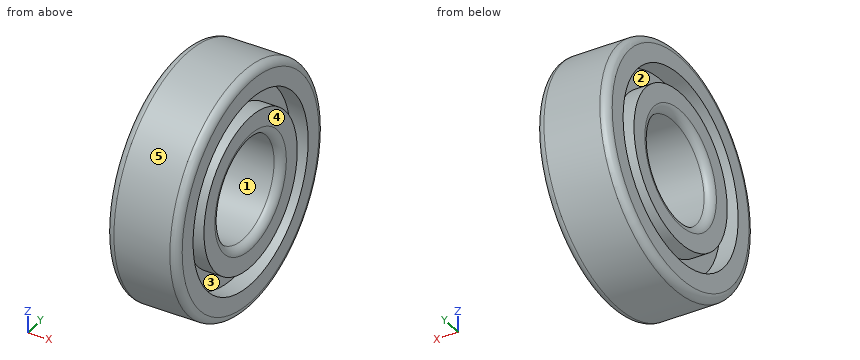
from build123d import *


with BuildPart() as part:
    # Эскиз1 → Повернуть1 (revolve)
    with BuildSketch(Plane.XY):
        with BuildLine():
            Line((5.5, 10), (-5.5, 10))
            ThreePointArc((-5.5, 10), (-6.560660172, 10.439339828), (-7, 11.5))
            Line((-7, 11.5), (-7, 15))
            Line((-7, 15), (-3.5, 15))
            Line((-3.5, 15), (-3.5, 18.5))
            Line((-3.5, 18.5), (-7, 18.5))
            Line((-7, 18.5), (-7, 22))
            ThreePointArc((-7, 22), (-6.560660172, 23.060660172), (-5.5, 23.5))
            Line((-5.5, 23.5), (5.5, 23.5))
            ThreePointArc((5.5, 23.5), (6.560660172, 23.060660172), (7, 22))
            Line((7, 22), (7, 18.5))
            Line((7, 18.5), (3.5, 18.5))
            Line((3.5, 18.5), (3.5, 15))
            Line((3.5, 15), (7, 15))
            Line((7, 15), (7, 11.5))
            ThreePointArc((7, 11.5), (6.560660172, 10.439339828), (5.5, 10))
        make_face()
    revolve(axis=Axis((-873.991742101, 0, 0), (1, 0, 0)))


solid = part.part
The listing builds one solid part. Answer for the finished solid, in the listing's coordinates (mm). Face numbers are marked on the shaded views. A direction names the side the tool comes from. Coordinates: 2 decimals unless noted, no trailing zeros. Order: outer loops, then holes, each group sorted by start corner. A loop starts at its lowest first (then second) coordinate and runs counter-clockwise, first axis right, second up.
Q1. Given P1, Ø22, axis at y = 0, z = 0, coming from the -X side; P2, Ø8, axis at x = -4, y = -14, coming from the +Z side; P3, Ø5, axis at x = 5.5, z = 13.5, coming from the +Y side, each flat-ended and moving along its own axis, determine where each tip first touches the part or whether it passes through.
Q2. For a pull along Y with two mould halves and no side action, classify the marked faces 3, 4 and 5 as pulls with the +Y half, pulls with the -Y half, needs draft (parallel to the pull), parting line crosses it, or undercut.
Q3. A cutting plane is placed at C-C, the plane x = 2.25. Write down the section's boundary in (y, z).
Q4. Consider line 1 (Z direction, x = -4.5, y = 0); line 2 (Z direction, x = 1, y = 0); line 3 (Y direction, x = -5.5, z = 10.5). Determine where each line is inside the solid, lowest interval first.
Q5. Which of the six approach directions +Z, -Z, +X, -X, +Y, -Y give full straight-line access (tool end or side, diameter ignored) to the marked faces 1 and 2?
Answers follow:
1. P1: stops at x = -6.91
1. P2: stops at z = 21.27
1. P3: stops at y = 20.77
2. face 3: undercut
2. face 4: needs draft
2. face 5: parting line crosses it
3. outline: circle Ø47 at (0, 0); hole circle Ø20 at (0, 0)
4. line 1: z = -23.5 to -18.5, -15 to -10, 10 to 15, 18.5 to 23.5
4. line 2: z = -23.5 to -10, 10 to 23.5
4. line 3: y = -21.02 to -15.23, -10.71 to 10.71, 15.23 to 21.02
5. face 1: +X, -X
5. face 2: -X
